Verification items for the finished model (mm, model axes). Face numbers are marked on the shaded views. Give positions to 0.01 mm unless a question says otherwise; leave off trailing zeros. Write each loop counter-clockwise with the first axis right and the second up, starting at its lowest first coordinate (ties: lowest second). Pieces come first, ordered by that corner, then holes.
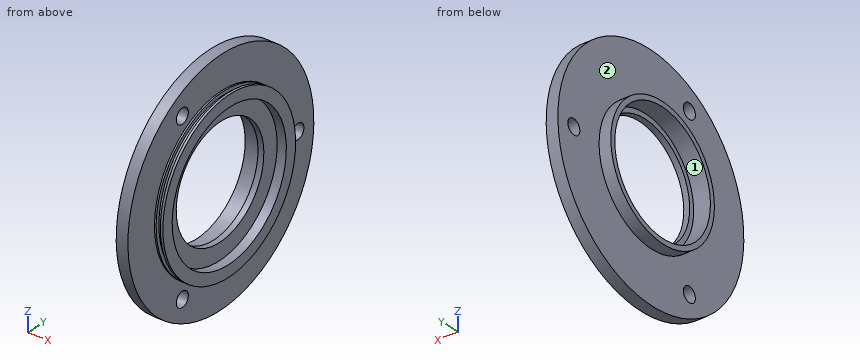
from build123d import *

# Parameters (mm, degrees)
SCHIZZO2_R               = 4.5
TAGLIO_ESTRUSIONE2_DEPTH = 57


with BuildPart() as part:
    # Schizzo1 → Rivoluzione1 (revolve)
    with BuildSketch(Plane.XY, mode=Mode.PRIVATE) as rivoluzione1_sk:
        Polygon((0, 43), (0, 50), (-1.5, 50), (-1.5, 47.95), (-4, 47.95), (-4, 50), (-5, 50), (-5, 70), (-12, 70), (-12, 39), (-19, 39), (-19, 36), (-9, 36), (-9, 33), (-5.5, 33), (-5.5, 43), align=None)
    revolve(rivoluzione1_sk.sketch.rotate(Axis((-54.554939241, 0, 0), (1, 0, 0)), 90), axis=Axis((-54.554939241, 0, 0), (1, 0, 0)))

    # Schizzo2 → Taglio-Estrusione2 (cut)
    with BuildSketch(Plane.ZY.offset(12)):
        with Locations((0, 58)):
            Circle(SCHIZZO2_R)
        with Locations((50.22947342, -29)):
            Circle(SCHIZZO2_R)
        with Locations((-50.229473419, -29)):
            Circle(SCHIZZO2_R)
    extrude(amount=-TAGLIO_ESTRUSIONE2_DEPTH, mode=Mode.SUBTRACT)


solid = part.part
Item 1: Scan lines: line 1 along Y through (x, z) = (-7.25, 0); line 2 along Y through (x, z) = (-3.05, 0); line 3 along X through (y, z) = (26.5, -25). Record each from-to range of solid material in increasing order.
Answer key:
line 1: y = -70 to -33, 33 to 53.5, 62.5 to 70
line 2: y = -47.95 to -43, 43 to 47.95
line 3: x = -19 to -5.5
Item 2: Sectioned sample at D-D on y = 58. Record the cut outline in (x, z).
Answer key:
outline: (-12, -39.19) - (-5, -39.19) - (-5, -4.5) - (-12, -4.5) - close; (-12, 4.5) - (-5, 4.5) - (-5, 39.19) - (-12, 39.19) - close
Item 3: Sectioned sample at C-C on z = 0. State how many separate pieces and enclosed holes the cut face has, then the cut area to 3 significant figures.
Answer key:
separate pieces: 3
enclosed holes: 0
area: 529 mm2
Item 4: Release check for a two-part mould opening along Z. For the marked faces 1 and 2 record: released by +Z, released by -Z, zero draft, split by the parting line, or undercut.
Answer key:
face 1: undercut
face 2: zero draft
Item 5: Depth check by flat-ended pin: pin 1 (1 mm diameter, centred on y = 23.5, z = 51.5, fed in from -X); pin 2 (14.5 mm diameter, centred on y = -29, z = -50.23, fed in from +X); pin 3 (3 mm diameter, centred on x = -12.5, z = -38.5, fed in from +Y); pin 4 (21.5 mm diameter, centred on y = -12, z = 17.5, fed in from -X). Enter the tip coordinate at first touch or a pass-through.
Answer key:
pin 1: stops at x = -12
pin 2: stops at x = -5
pin 3: stops at y = 59.37
pin 4: passes through
